The model under review builds one solid part; all positions refer to its coordinate system, in mm. Face numbers are marked on the shaded views. A direction names the side the tool comes from. Give positions to 0.01 mm unless a question says otherwise; leave off trailing zeros. Order: outer loops, then holes, each group sorted by start corner. A loop starts at its lowest first (then second) coordinate and runs counter-clockwise, first axis right, second up.
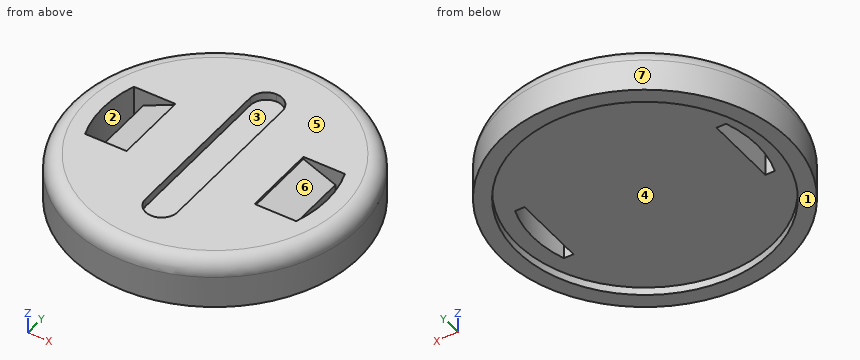
```python
from build123d import *

# Parameters (mm, degrees)
SKETCH_1_R          = 9
EXTRUDE_1_DEPTH     = 3
FILLET_1_R          = 1
SKETCH_3_W          = 2
SKETCH_3_H          = 12
CUT_EXTRUDE_1_DEPTH = 0.5
FILLET_2_R          = 1
CUT_EXTRUDE_2_DEPTH = 1
CHAMFER_2_SIZE      = 2
CHAMFER_2_SIZE2     = 0.932615316
CHAMFER_5_SIZE      = 2
CHAMFER_5_SIZE2     = 0.848949632
CUT_EXTRUDE_3_DEPTH = 8
CUT_EXTRUDE_START   = -2
SKETCH_7_R          = 7
CUT_EXTRUDE_4_DEPTH = 2
EXTRUDE_2_DEPTH     = 2
SKETCH_9_R          = 8
CUT_EXTRUDE_5_DEPTH = 0.5


with BuildPart() as part:
    # 草图1 → 凸台-拉伸1 (new body)
    with BuildSketch(Plane(origin=(0, 0, 12), x_dir=(-1, 0, 0), z_dir=(0, 0, -1))):
        Circle(SKETCH_1_R)
    extrude(amount=-EXTRUDE_1_DEPTH)

    # 圆角1
    fillet_1_edges = [part.edges().sort_by_distance(p)[0] for p in [
        (9, 0, 15),
    ]]
    fillet(fillet_1_edges, radius=FILLET_1_R)

    # 草图3 → 切除-拉伸1 (cut)
    with BuildSketch(Plane.XY.offset(15)):
        with Locations((0, -0.105406486)):
            Rectangle(SKETCH_3_W, SKETCH_3_H)
    extrude(amount=-CUT_EXTRUDE_1_DEPTH, mode=Mode.SUBTRACT)

    # 圆角2
    fillet_2_edges = [part.edges().sort_by_distance(p)[0] for p in [
        (1, -6.105406486, 14.75),
        (-1, -6.105406486, 14.75),
        (1, 5.894593514, 14.75),
        (-1, 5.894593514, 14.75),
    ]]
    fillet(fillet_2_edges, radius=FILLET_2_R - 0.0001)  # a hair under: the kernel refuses the full size

    # 草图4 → 切除-拉伸2 (cut)
    with BuildSketch(Plane.XY.offset(15)):
        with BuildLine():
            Line((-6.599663291, 2.333333333), (-4, 2.333333333))
            Line((-4, 2.333333333), (-4, -2.333333333))
            Line((-4, -2.333333333), (-6.599663291, -2.333333333))
            ThreePointArc((-6.599663291, -2.333333333), (-7, 0), (-6.599663291, 2.333333333))
        make_face()
        with BuildLine():
            Line((4, -2.333333333), (6.599663291, -2.333333333))
            ThreePointArc((6.599663291, -2.333333333), (7, 0), (6.599663291, 2.333333333))
            Line((6.599663291, 2.333333333), (4, 2.333333333))
            Line((4, 2.333333333), (4, -2.333333333))
        make_face()
    extrude(amount=-CUT_EXTRUDE_2_DEPTH, mode=Mode.SUBTRACT)

    # 倒角2
    chamfer_2_edges = [part.edges().sort_by_distance(p)[0] for p in [
        (-4, 0, 14),
    ]]
    chamfer_2_side = [part.faces().sort_by_distance(p)[0] for p in [
        (-5.436521823, 0, 14),
    ]]
    chamfer(chamfer_2_edges, length=CHAMFER_2_SIZE, length2=CHAMFER_2_SIZE2, reference=chamfer_2_side[0])

    # 倒角5
    chamfer_5_edges = [part.edges().sort_by_distance(p)[0] for p in [
        (4, 0, 14),
    ]]
    chamfer_5_side = [part.faces().sort_by_distance(p)[0] for p in [
        (5.436521823, 0, 14),
    ]]
    chamfer(chamfer_5_edges, length=CHAMFER_5_SIZE, length2=CHAMFER_5_SIZE2, reference=chamfer_5_side[0])

    # 草图6 → 切除-拉伸3 (cut)
    with BuildSketch(Plane.XY.offset(14)):
        with BuildLine():
            Line((-6.599663291, -2.333333333), (-6, -2.333333333))
            Line((-6, -2.333333333), (-6, 2.333333333))
            Line((-6, 2.333333333), (-6.599663291, 2.333333333))
            ThreePointArc((-6.599663291, 2.333333333), (-7, 0), (-6.599663291, -2.333333333))
        make_face()
        with BuildLine():
            Line((6.599663291, 2.333333333), (6, 2.333333333))
            Line((6, 2.333333333), (6, -2.333333333))
            Line((6, -2.333333333), (6.599663291, -2.333333333))
            ThreePointArc((6.599663291, -2.333333333), (7, 0), (6.599663291, 2.333333333))
        make_face()
    extrude(amount=-CUT_EXTRUDE_3_DEPTH, mode=Mode.SUBTRACT)

    # 草图7 → 切除-拉伸4 (cut)
    with BuildSketch(Plane(origin=(0, 0, 12), x_dir=(-1, 0, 0), z_dir=(0, 0, -1)).offset(CUT_EXTRUDE_START)):
        with Locations(Location((0, 0, 0), (0, 0, 199.471220634))):
            Circle(SKETCH_7_R)
    extrude(amount=CUT_EXTRUDE_4_DEPTH, mode=Mode.SUBTRACT)

    # 草图8 → 凸台-拉伸2 (add)
    with BuildSketch(Plane(origin=(0, 0, 14), x_dir=(-1, 0, 0), z_dir=(0, 0, -1))):
        with BuildLine():
            Line((-6.599663291, 2.333333333), (-6, 2.333333333))
            Line((-6, 2.333333333), (-6, -2.333333333))
            Line((-6, -2.333333333), (-6.599663291, -2.333333333))
            ThreePointArc((-6.599663291, -2.333333333), (0, -7), (6.599663291, -2.333333333))
            Line((6.599663291, -2.333333333), (6, -2.333333333))
            Line((6, -2.333333333), (6, 2.333333333))
            Line((6, 2.333333333), (6.599663291, 2.333333333))
            ThreePointArc((6.599663291, 2.333333333), (0, 7), (-6.599663291, 2.333333333))
        make_face()
    extrude(amount=EXTRUDE_2_DEPTH)

    # 草图9 → 切除-拉伸5 (cut)
    with BuildSketch(Plane(origin=(0, 0, 12), x_dir=(-1, 0, 0), z_dir=(0, 0, -1))):
        Circle(SKETCH_9_R)
    extrude(amount=-CUT_EXTRUDE_5_DEPTH, mode=Mode.SUBTRACT)


solid = part.part
```
Item 1: Take a section at A-A (z = 12.95). Give the boundary of the cut face in (x, y).
Values found:
outline: circle Ø18 at (0, 0); hole (-6.6, -2.33) - (-6, -2.33) - (-6, 2.33) - (-6.6, 2.33) arc R7 ccw to start; hole (6, -2.33) - (6.6, -2.33) arc R7 ccw to (6.6, 2.33) - (6, 2.33) - close
Item 2: Take a section at B-B (y = 0). Give the boundary of the cut face in (x, z).
Values found:
outline: (-9, 12) - (-8, 12) - (-8, 12.5) - (-7, 12.5) - (-7, 15) - (-8, 15) arc R1 ccw to (-9, 14) - close; (-6, 12.5) - (6, 12.5) - (6, 14) - (4, 14.85) - (4, 15) - (1, 15) - (1, 14.5) - (-1, 14.5) - (-1, 15) - (-4, 15) - (-4, 14.93) - (-6, 14) - close; (7, 12.5) - (8, 12.5) - (8, 12) - (9, 12) - (9, 14) arc R1 ccw to (8, 15) - (7, 15) - close
Item 3: For the marked faces 1, 2 and 3, list the 3-axis set-ups (+Z, -Z, +X, -X, +Y, -Y) from which the entire face can be reached by the end or side of a thin tool; tool diameter is ignored.
Values found:
face 1: -Z, +X, -X, +Y, -Y
face 2: +Z, -Z
face 3: +Z
Item 4: Clearance check with flat-ended pins moving along their axes: pin 1 Ø8 at (x, y) = (5.5, 4.5) entering from -Z; pin 2 Ø1.5 at (x, z) = (5.5, 13) entering from -Y; pin 3 Ø1.2 at (x, z) = (6, 14) entering from -Y; pin 4 Ø1.6 at (x, y) = (0, 2.5) entering from +Z. State where each tip first meets the part, or that it passes through.
Values found:
pin 1: stops at z = 12
pin 2: stops at y = -7.64
pin 3: stops at y = -7.2
pin 4: stops at z = 14.5
Item 5: For line 1 (Y direction, x = 0, z = 12.2); line 2 (X direction, y = 1.5, z = 13.15); line 3 (X direction, y = -5, z = 14.8), list the stretches that pass through material, from the lowest coordinate up.
Values found:
line 1: y = -9 to -8, 8 to 9
line 2: x = -8.87 to -6.84, -6 to 6, 6.84 to 8.87
line 3: x = -7 to -1, 1 to 7
Item 6: Draft analysis for pull direction Y (two halves, no side actions). For the marked faces 4, 5, 6 and 7, state which applies: released by +Y, released by -Y, zero draft, split by the parting line, or undercut.
Values found:
face 4: undercut
face 5: zero draft
face 6: undercut
face 7: split by the parting line
